CAD build for the part. Positions are in the model's coordinates, mm. Round coordinates to 2 decimals unless told otherwise and drop trailing zeros. Write each loop counter-clockwise with the first axis right and the second up, starting at its lowest first coordinate (ties: lowest second). Pieces come first, ordered by that corner, then holes. Notation, with made-up numbers: (20, 5.5) - (77, 5.5) arc R15 ccw to (77, 24.5) - close; hole circle Ø5 at (-20, 38.25). An arc over 180 degrees is marked (long way). Put each result on its own line as item: value. Start each with the question number.
Item 1: Drill centre lines: line 1 (X direction, y = 10.75, z = 0); line 2 (Y direction, x = -5, z = 27); line 3 (X direction, y = 8.5, z = -2.5). Where is each one in solid material? Low to high. Write a range as from..to.
Item 2: Pin check, flat tips, straight feed: pin 1 Ø8 at (x, y) = (-21, 8.5) entering from +Z; pin 2 Ø4 at (x, y) = (-30, 23) entering from +Z; pin 3 Ø1.5 at (x, y) = (-35.5, 16) entering from -Z. Stop position of each tip, or through.
Item 3: Cut at C-C (y = 6.5). Give the cut face in (x, z).
Item 4: Cut at D-D (y = 42.5). Give the cut face in (x, z), and give its area (3 significant figures).
Item 5: Cut at B-B (x = 0). Give the cut face in (y, z), and give its area (3 significant figures).
Item 6: Mould opens along Z. For faces 1 (the flat face through (1, 50, -1)), 2 (the cylindrical face through (1.32, 14.79, 29.97)), 3 (the flat face through (0, 30, 0)), 4 (the cylindrical face through (15.02, 24.65, 47.69)) say: released by +Z, released by -Z, zero draft, split by the parting line, or undercut.
Item 7: Cut at A-A (z = 0). Give the cut face in (x, y).
```python
from build123d import *

# Parameters (mm, degrees)
SKETCH1_W           = 50
SKETCH1_H           = 25
BOSS_EXTRUDE1_DEPTH = 25
FILLET2_R           = 5
CUT_EXTRUDE1_DEPTH  = 15
SKETCH3_R           = 50
BOSS_EXTRUDE2_DEPTH = 50
SKETCH4_R           = 30
CUT_EXTRUDE2_DEPTH  = 30


with BuildPart() as part:
    # Sketch1 → Boss-Extrude1 (new body)
    with BuildSketch(Plane(origin=(0, 0, 0), x_dir=(1, 0, 0), z_dir=(0, 1, 0))):
        Rectangle(SKETCH1_W, SKETCH1_H)
    extrude(amount=BOSS_EXTRUDE1_DEPTH)

    # Fillet2
    fillet2_edges = [part.edges().sort_by_distance(p)[0] for p in [
        (25, 12.5, 12.5),
        (-25, 12.5, 12.5),
        (-25, 12.5, -12.5),
        (25, 12.5, -12.5),
    ]]
    fillet(fillet2_edges, radius=FILLET2_R)

    # Sketch2 → Cut-Extrude1 (cut)
    with BuildSketch(Plane(origin=(0, 25, 0), x_dir=(1, 0, 0), z_dir=(0, 1, 0))):
        with BuildLine():
            Line((-13.058351702, 9.034247402), (13.06, 9.034247402))
            ThreePointArc((13.06, 9.034247402), (22.094247402, 0), (13.06, -9.034247402))
            Line((13.06, -9.034247402), (-13.058351702, -9.034247402))
            ThreePointArc((-13.058351702, -9.034247402), (-22.092599103, 0), (-13.058351702, 9.034247402))
        make_face()
    extrude(amount=-CUT_EXTRUDE1_DEPTH, mode=Mode.SUBTRACT)

    # Sketch3 → Boss-Extrude2 (add)
    with BuildSketch(Plane(origin=(0, 0, 0), x_dir=(1, 0, 0), z_dir=(0, 1, 0))):
        with Locations(Location((0, 0, 0), (0, 0, 270))):
            Circle(SKETCH3_R)
    extrude(amount=BOSS_EXTRUDE2_DEPTH)

    # Sketch4 → Cut-Extrude2 (cut)
    with BuildSketch(Plane.XZ):
        with Locations(Location((0, 0, 0), (0, 0, 270))):
            Circle(SKETCH4_R)
    extrude(amount=-CUT_EXTRUDE2_DEPTH, mode=Mode.SUBTRACT)


solid = part.part
```
Output values:
1. line 1: -50..-30, 30..50
1. line 2: 30..50
1. line 3: -49.94..-29.9, 29.9..49.94
2. pin 1: z = 47.02
2. pin 2: z = 41.42
2. pin 3: z = -35.95
3. outline: circle Ø100 at (0, 0); hole circle Ø60 at (0, 0)
4. outline: circle Ø100 at (0, 0)
4. area: 7,850 mm2
5. outline: (0, -50) - (50, -50) - (50, 50) - (0, 50) - (0, 30) - (30, 30) - (30, -30) - (0, -30) - close
5. area: 3,200 mm2
6. face 1: zero draft
6. face 2: undercut
6. face 3: undercut
6. face 4: split by the parting line
7. outline: (-50, 0) - (-30, 0) - (-30, 30) - (30, 30) - (30, 0) - (50, 0) - (50, 50) - (-50, 50) - close
